Input: part model. Units: mm. Frame: model coordinates. A direction names the side the tool comes from. Coordinates: 2 decimals unless noted, no trailing zeros. Loops run counter-clockwise (first coordinate to the right, second up) from the corner with the lowest first, then second, coordinate; pieces in that order, holes last.
```python
from build123d import *

# Parameters (mm, degrees)
F0_W     = 25
F0_H     = 23.2
F0_R     = 9
F1_DEPTH = 2
F2_DEPTH = 12.5
F4_DEPTH = 4
F5_R     = 1
F5_R_2   = 4.5
F6_DEPTH = 2


with BuildPart() as f1:
    # F0 (on Top) → F1 (new body)
    with BuildSketch(Plane.XY):
        Rectangle(F0_W, F0_H)
        Polygon((10, 10), (10, 0), (10, -10), (0, -10), (-10, -10), (-10, 0), (-10, 10), (0, 10), align=None, mode=Mode.SUBTRACT)
        with BuildLine():
            ThreePointArc((0, -10), (7.0710678119, -7.0710678119), (10, 0))
            ThreePointArc((10, 0), (7.0710678119, 7.0710678119), (0, 10))
            ThreePointArc((0, 10), (-7.0710678119, 7.0710678119), (-10, 0))
            ThreePointArc((-10, 0), (-7.0710678119, -7.0710678119), (0, -10))
        make_face()
        Circle(F0_R, mode=Mode.SUBTRACT)
        with BuildLine():
            Line((-10, -10), (0, -10))
            ThreePointArc((0, -10), (-7.0710678119, -7.0710678119), (-10, 0))
            Line((-10, 0), (-10, -10))
        make_face()
        with BuildLine():
            ThreePointArc((-10, 0), (-7.0710678119, 7.0710678119), (0, 10))
            Line((0, 10), (-10, 10))
            Line((-10, 10), (-10, 0))
        make_face()
        with BuildLine():
            ThreePointArc((0, 10), (7.0710678119, 7.0710678119), (10, 0))
            Line((10, 0), (10, 10))
            Line((10, 10), (0, 10))
        make_face()
        with BuildLine():
            Line((10, -10), (10, 0))
            ThreePointArc((10, 0), (7.0710678119, -7.0710678119), (0, -10))
            Line((0, -10), (10, -10))
        make_face()
    extrude(amount=-F1_DEPTH)

    # F0 (on Top) → F2 (join)
    with BuildSketch(Plane.XY):
        Rectangle(F0_W, F0_H)
        Polygon((10, 10), (10, 0), (10, -10), (0, -10), (-10, -10), (-10, 0), (-10, 10), (0, 10), align=None, mode=Mode.SUBTRACT)
    extrude(amount=F2_DEPTH)

    # F3 (on face) → F4 (cut)
    with BuildSketch(Plane(origin=(0, 11.6, 0), x_dir=(-1, 0, 0), z_dir=(0, 1, 0))):
        with BuildLine():
            ThreePointArc((0, 9.1), (-0.7778174593, 7.2221825407), (1.1, 8))
            ThreePointArc((1.1, 8), (0.7778174593, 8.7778174593), (0, 9.1))
        make_face()
    extrude(amount=-F4_DEPTH, mode=Mode.SUBTRACT)

    # F5 (on face) → F6 (join)
    with BuildSketch(Plane.XY.offset(12.5)):
        Polygon((-12.5, 11.6), (-12.5, -11.6), (12.5, -11.6), (12.5, 15.6), (-12.5, 15.6), align=None)
        with Locations((-10.16, 0)):
            Circle(F5_R, mode=Mode.SUBTRACT)
        Circle(F5_R_2, mode=Mode.SUBTRACT)
        with Locations((10.16, 0)):
            Circle(F5_R, mode=Mode.SUBTRACT)
    extrude(amount=F6_DEPTH)


solid = f1.part
```
Item 1: Mould query, pull axis X, two halves, no side actions, for faces 1 (the face through (0, 5, 14.5)), 2 (the face through (-12.5, 2, 6)), 3 (the face through (9.37, -0.61, 13.49)). Classes: +X half, -X half, draft (parallel to the pull), parting line (faces both ways), or undercut.
Result:
face 1: draft
face 2: -X half
face 3: undercut
Item 2: Line query: L1, parallel to Y at x = 0, z = 13.1; L2, parallel to Y at x = -9, z = 6.5; L3, parallel to X at y = 11.1, z = 8. Output: solid intervals per line, ascending.
Result:
L1: y = -11.6 to -4.5, 4.5 to 15.6
L2: y = -11.6 to -10, 10 to 11.6
L3: x = -12.5 to -1.1, 1.1 to 12.5
Item 3: Section query D-D (z = 7.5). Output: boundary loops of the cut face in (x, y).
Result:
outline: (-12.5, -11.6) - (12.5, -11.6) - (12.5, 11.6) - (0.98, 11.6) - (0.98, 10) - (10, 10) - (10, -10) - (-10, -10) - (-10, 10) - (-0.98, 10) - (-0.98, 11.6) - (-12.5, 11.6) - close
Item 4: Section query B-B (x = 3.75). Output: boundary loops of the cut face in (y, z).
Result:
outline: (-11.6, -2) - (-8.18, -2) - (-8.18, 0) - (-10, 0) - (-10, 12.5) - (-2.49, 12.5) - (-2.49, 14.5) - (-11.6, 14.5) - close; (2.49, 12.5) - (10, 12.5) - (10, 0) - (8.18, 0) - (8.18, -2) - (11.6, -2) - (11.6, 12.5) - (15.6, 12.5) - (15.6, 14.5) - (2.49, 14.5) - close
Item 5: Section query A-A (y = 0). Output: boundary loops of the cut face in (x, z), then the cut area to 4 significant figures.
Result:
outline: (-12.5, -2) - (-9, -2) - (-9, 0) - (-10, 0) - (-10, 12.5) - (-11.16, 12.5) - (-11.16, 14.5) - (-12.5, 14.5) - close; (-9.16, 12.5) - (-4.5, 12.5) - (-4.5, 14.5) - (-9.16, 14.5) - close; (4.5, 12.5) - (9.16, 12.5) - (9.16, 14.5) - (4.5, 14.5) - close; (9, -2) - (12.5, -2) - (12.5, 14.5) - (11.16, 14.5) - (11.16, 12.5) - (10, 12.5) - (10, 0) - (9, 0) - close
area: 100.5 mm2
Item 6: Reachability of faces 4 (the face through (10.4, 0, 12.5)), 5 (the face through (-2, 9, 0)), 6 (the face through (0, 14, 12.5)) from +Z, -Z, +X, -X, +Y, -Y: full face, straight path, thin tool, end or side. Return the list, or none.
Result:
face 4: +Z
face 5: none
face 6: -Z, +X, -X, +Y
Item 7: Section query C-C (z = -0.75). Output: boundary loops of the cut face in (x, y), then the cut area to 3 significant figures.
Result:
outline: (-12.5, -11.6) - (12.5, -11.6) - (12.5, 11.6) - (-12.5, 11.6) - close; hole circle Ø18 at (0, 0)
area: 326 mm2
Item 8: Contact query for flat-ended pins moving along their axis: P1, Ø5, axis at x = -4.5, z = 4, coming from the +Y side; P2, Ø14.5, axis at x = 0, y = 0, coming from the -Z side. Output: stop coordinate, or through.
Result:
P1: stops at y = 11.6
P2: stops at z = 12.5
